The model under review builds one solid part; all positions refer to its coordinate system, in mm. A direction names the side the tool comes from. Coordinates: 2 decimals unless noted, no trailing zeros. Loops run counter-clockwise (first coordinate to the right, second up) from the corner with the lowest first, then second, coordinate; pieces in that order, holes last. Notation, with made-up numbers: M 33.5,46.5 L 56.5,46.5 A25 ccw 56.5,62.5 Z; hole C -5,-32 d5. An arc over 180 degrees is marked long. Return JSON: item names as keys, results as strings.
```python
from build123d import *

# Parameters (mm, degrees)
SKETCH1_R           = 2.54
BOSS_EXTRUDE1_DEPTH = 2.286
FILLET1_R           = 6.35


with BuildPart() as part:
    # Sketch1 → Boss-Extrude1 (new body)
    with BuildSketch(Plane(origin=(0, 0, 0), x_dir=(1, 0, 0), z_dir=(0, 1, 0))):
        Polygon((25.4, 114.3), (0, 114.3), (0, 0), (25.4, 0), (25.4, 31.75), (69.85, 31.75), (69.85, 82.55), (25.4, 82.55), align=None)
        with Locations(Location((12.7, 95.25, 0), (0, 0, 270))):
            Circle(SKETCH1_R, mode=Mode.SUBTRACT)
        with Locations(Location((12.7, 69.85, 0), (0, 0, 270))):
            Circle(SKETCH1_R, mode=Mode.SUBTRACT)
        with Locations(Location((12.7, 44.45, 0), (0, 0, 270))):
            Circle(SKETCH1_R, mode=Mode.SUBTRACT)
        with Locations(Location((12.7, 19.05, 0), (0, 0, 270))):
            Circle(SKETCH1_R, mode=Mode.SUBTRACT)
        with Locations(Location((38.1, 69.85, 0), (0, 0, 270))):
            Circle(SKETCH1_R, mode=Mode.SUBTRACT)
        with Locations(Location((50.8, 69.85, 0), (0, 0, 270))):
            Circle(SKETCH1_R, mode=Mode.SUBTRACT)
        with Locations(Location((63.5, 69.85, 0), (0, 0, 270))):
            Circle(SKETCH1_R, mode=Mode.SUBTRACT)
        with Locations(Location((50.8, 57.15, 0), (0, 0, 270))):
            Circle(SKETCH1_R, mode=Mode.SUBTRACT)
        with Locations(Location((63.5, 57.15, 0), (0, 0, 270))):
            Circle(SKETCH1_R, mode=Mode.SUBTRACT)
        with Locations(Location((50.8, 44.45, 0), (0, 0, 270))):
            Circle(SKETCH1_R, mode=Mode.SUBTRACT)
        with Locations(Location((63.5, 44.45, 0), (0, 0, 270))):
            Circle(SKETCH1_R, mode=Mode.SUBTRACT)
        with Locations(Location((38.1, 57.15, 0), (0, 0, 270))):
            Circle(SKETCH1_R, mode=Mode.SUBTRACT)
        with Locations(Location((38.1, 44.45, 0), (0, 0, 270))):
            Circle(SKETCH1_R, mode=Mode.SUBTRACT)
    extrude(amount=BOSS_EXTRUDE1_DEPTH)

    # Fillet1
    fillet1_edges = [part.edges().sort_by_distance(p)[0] for p in [
        (25.4, 1.143, -82.55),
        (69.85, 1.143, -82.55),
        (69.85, 1.143, -31.75),
        (25.4, 1.143, -31.75),
        (25.4, 1.143, 0),
        (0, 1.143, 0),
        (0, 1.143, -114.3),
        (25.4, 1.143, -114.3),
    ]]
    fillet(fillet1_edges, radius=FILLET1_R)


solid = part.part
```
1. Insertion check: pin 1 Ø1.1 at (y, z) = (1.5, -95.5) entering from +X; pin 2 Ø4 at (x, z) = (63.5, -57.15) entering from +Y; pin 3 Ø0.7 at (x, y) = (47, 0.5) entering from -Z. Each pin has a flat end and moves straight along its axis. Give the tip position at first contact, or say it passes through.
Check values:
{"pin 1": "x = 25.4", "pin 2": "through", "pin 3": "z = -82.55"}
2. To check wall thickness, follow line 1 (X direction, y = 0.95, z = -57.15); line 2 (X direction, y = 0.5, z = -69.85); line 3 (X direction, y = 0.6, z = -95.25). State the ranges of each line that lie inside material, in increasing order.
Check values:
{"line 1": "0 to 35.56, 40.64 to 48.26, 53.34 to 60.96, 66.04 to 69.85", "line 2": "0 to 10.16, 15.24 to 35.56, 40.64 to 48.26, 53.34 to 60.96, 66.04 to 69.85", "line 3": "0 to 10.16, 15.24 to 25.4"}
3. Add section C-C on z = -44.45. Give the boundary of the cut face in (x, y).
Check values:
{"outline": "M 0,0 L 10.16,0 L 10.16,2.29 L 0,2.29 Z; M 15.24,0 L 35.56,0 L 35.56,2.29 L 15.24,2.29 Z; M 40.64,0 L 48.26,0 L 48.26,2.29 L 40.64,2.29 Z; M 53.34,0 L 60.96,0 L 60.96,2.29 L 53.34,2.29 Z; M 66.04,0 L 69.85,0 L 69.85,2.29 L 66.04,2.29 Z"}
4. Machinability: for faces 1 (the face through (25.4, 1, -16)), 2 (the face through (40.24, 1.13, -43.08)), 3 (the face through (25.4, 1, -98)), which of the approach directions +Z, -Z, +X, -X, +Y, -Y give a long, thin tool a straight path to every point of the face, cutting with its end or side? Answer none if there is none.
Check values:
{"face 1": "+Z, +X, +Y, -Y", "face 2": "+Y, -Y", "face 3": "-Z, +X, +Y, -Y"}
5. Add section A-A on x = 12.7. Give the boundary of the cut face in (y, z), plus the area to 3 significant figures.
Check values:
{"outline": "M 0,-114.3 L 2.29,-114.3 L 2.29,-97.79 L 0,-97.79 Z; M 0,-92.71 L 2.29,-92.71 L 2.29,-72.39 L 0,-72.39 Z; M 0,-67.31 L 2.29,-67.31 L 2.29,-46.99 L 0,-46.99 Z; M 0,-41.91 L 2.29,-41.91 L 2.29,-21.59 L 0,-21.59 Z; M 0,-16.51 L 2.29,-16.51 L 2.29,0 L 0,0 Z", "area": "215 mm²"}
6. Add section D-D on y = 1.8. State how many separate pieces and enclosed holes the cut face has, plus the area to 3 significant figures.
Check values:
{"separate pieces": "1", "enclosed holes": "13", "area": "4,860 mm²"}
7. Add section B-B on x = 50.8. Give the boundary of the cut face in (y, z), plus the area to 3 significant figures.
Check values:
{"outline": "M 0,-82.55 L 2.29,-82.55 L 2.29,-72.39 L 0,-72.39 Z; M 0,-67.31 L 2.29,-67.31 L 2.29,-59.69 L 0,-59.69 Z; M 0,-54.61 L 2.29,-54.61 L 2.29,-46.99 L 0,-46.99 Z; M 0,-41.91 L 2.29,-41.91 L 2.29,-31.75 L 0,-31.75 Z", "area": "81.3 mm²"}
8. The part is to be moulded in two halves that separate along Z. For faces 4 (the face through (68.04, 1.16, -33.66)), 5 (the face through (1.91, 1.16, -112.49)), 6 (the face through (27, 2.286, -58)), 7 (the face through (39.82, 1.13, -71.72)), say which applies: released by +Z, released by -Z, zero draft, split by the parting line, or undercut.
Check values:
{"face 4": "released by +Z", "face 5": "released by -Z", "face 6": "zero draft", "face 7": "undercut"}
